from build123d import *

# Parameters (mm, degrees)
SKETCH_1_R      = 1.75
SKETCH_1_W      = 3
SKETCH_1_H      = 8
SKETCH_1_W_2    = 41
SKETCH_1_H_2    = 11
EXTRUDE_1_DEPTH = 5


with BuildPart() as part:
    # Эскиз1 → Бобышка-Вытянуть1 (new body)
    with BuildSketch(Plane(origin=(0, 0, 0), x_dir=(0, 0, -1), z_dir=(1, 0, 0))):
        with BuildLine():
            Line((-36.75, 45), (-36.75, 42.5))
            Line((-36.75, 42.5), (-39.25, 42.5))
            Line((-39.25, 42.5), (-39.25, 40))
            Line((-39.25, 40), (-30.75, 40))
            Line((-30.75, 40), (-30.75, 42.5))
            Line((-30.75, 42.5), (-33.25, 42.5))
            Line((-33.25, 42.5), (-33.25, 45))
            Line((-33.25, 45), (33.25, 45))
            Line((33.25, 45), (33.25, 42.5))
            Line((33.25, 42.5), (30.75, 42.5))
            Line((30.75, 42.5), (30.75, 40))
            Line((30.75, 40), (39.25, 40))
            Line((39.25, 40), (39.25, 42.5))
            Line((39.25, 42.5), (36.75, 42.5))
            Line((36.75, 42.5), (36.75, 45))
            Line((36.75, 45), (43, 45))
            ThreePointArc((43, 45), (44.414213562, 44.414213562), (45, 43))
            Line((45, 43), (45, 31.75))
            Line((45, 31.75), (42.5, 31.75))
            Line((42.5, 31.75), (42.5, 34.25))
            Line((42.5, 34.25), (40, 34.25))
            Line((40, 34.25), (40, 25.75))
            Line((40, 25.75), (42.5, 25.75))
            Line((42.5, 25.75), (42.5, 28.25))
            Line((42.5, 28.25), (45, 28.25))
            Line((45, 28.25), (45, -28.25))
            Line((45, -28.25), (42.5, -28.25))
            Line((42.5, -28.25), (42.5, -25.75))
            Line((42.5, -25.75), (40, -25.75))
            Line((40, -25.75), (40, -34.25))
            Line((40, -34.25), (42.5, -34.25))
            Line((42.5, -34.25), (42.5, -31.75))
            Line((42.5, -31.75), (45, -31.75))
            Line((45, -31.75), (45, -43))
            ThreePointArc((45, -43), (44.414213562, -44.414213562), (43, -45))
            Line((43, -45), (36.75, -45))
            Line((36.75, -45), (36.75, -42.5))
            Line((36.75, -42.5), (39.25, -42.5))
            Line((39.25, -42.5), (39.25, -40))
            Line((39.25, -40), (30.75, -40))
            Line((30.75, -40), (30.75, -42.5))
            Line((30.75, -42.5), (33.25, -42.5))
            Line((33.25, -42.5), (33.25, -45))
            Line((33.25, -45), (-33.25, -45))
            Line((-33.25, -45), (-33.25, -42.5))
            Line((-33.25, -42.5), (-30.75, -42.5))
            Line((-30.75, -42.5), (-30.75, -40))
            Line((-30.75, -40), (-39.25, -40))
            Line((-39.25, -40), (-39.25, -42.5))
            Line((-39.25, -42.5), (-36.75, -42.5))
            Line((-36.75, -42.5), (-36.75, -45))
            Line((-36.75, -45), (-43, -45))
            ThreePointArc((-43, -45), (-44.414213562, -44.414213562), (-45, -43))
            Line((-45, -43), (-45, -31.75))
            Line((-45, -31.75), (-42.5, -31.75))
            Line((-42.5, -31.75), (-42.5, -34.25))
            Line((-42.5, -34.25), (-40, -34.25))
            Line((-40, -34.25), (-40, -25.75))
            Line((-40, -25.75), (-42.5, -25.75))
            Line((-42.5, -25.75), (-42.5, -28.25))
            Line((-42.5, -28.25), (-45, -28.25))
            Line((-45, -28.25), (-45, 28.25))
            Line((-45, 28.25), (-42.5, 28.25))
            Line((-42.5, 28.25), (-42.5, 25.75))
            Line((-42.5, 25.75), (-40, 25.75))
            Line((-40, 25.75), (-40, 34.25))
            Line((-40, 34.25), (-42.5, 34.25))
            Line((-42.5, 34.25), (-42.5, 31.75))
            Line((-42.5, 31.75), (-45, 31.75))
            Line((-45, 31.75), (-45, 43))
            ThreePointArc((-45, 43), (-44.414213562, 44.414213562), (-43, 45))
            Line((-43, 45), (-36.75, 45))
        make_face()
        with Locations((-30, -22.5)):
            Circle(SKETCH_1_R, mode=Mode.SUBTRACT)
        with Locations((30, -22.5)):
            Circle(SKETCH_1_R, mode=Mode.SUBTRACT)
        with Locations((8.5, -10)):
            Rectangle(SKETCH_1_W, SKETCH_1_H, mode=Mode.SUBTRACT)
        with Locations((-8.5, -10)):
            Rectangle(SKETCH_1_W, SKETCH_1_H, mode=Mode.SUBTRACT)
        with Locations((4.5, 14.5)):
            Rectangle(SKETCH_1_W_2, SKETCH_1_H_2, mode=Mode.SUBTRACT)
    extrude(amount=EXTRUDE_1_DEPTH)


solid = part.part
Work out the finished part from the listing and answer in its coordinate system (mm). A direction names the side the tool comes from. Give positions to 0.01 mm unless a question says otherwise; leave off trailing zeros. Order: outer loops, then holes, each group sorted by start corner. A loop starts at its lowest first (then second) coordinate and runs counter-clockwise, first axis right, second up. Notation, with made-up numbers: (-6.5, -13.75) - (5.5, -13.75) arc R16 cw to (5.5, -1.75) - close; hole circle Ø5 at (58.25, 10). An arc over 180 degrees is marked (long way). Answer as CSV lines item,"result". Start each with the question number.
Q1. Find the intervals of material crossed by L1, parallel to Z at x = 1.3, y = -13.5; L2, parallel to Z at x = 0.55, y = 33.5, in increasing order. Write a range as [from, to].
Q2. For faces 4 (the face through (2, 44, 36.75)), 5 (the face through (2, 31.75, -44)), 6 (the face through (2, -44, 33.25)), 7 (the face through (2, 14, 16)), determine the directions among +Z, -Z, +X, -X, +Y, -Y from which every point of the face is accessible in a straight line to the end or side of a thin tool.
Q3. The part is cut by section D-D (y = 30). Write down the section's boundary in (x, z), then the cut area to 3 significant figures.
Q4. The part is cut by section B-B (z = -18.5). Write down the section's boundary in (x, y).
Q5. The part is cut by section C-C (x = 1.2). Give the number of separate pieces and of enclosed holes in the cut face, then the cut area to 3 significant figures.
Q6. The part is cut by section A-A (y = -22.5). Write down the section's boundary in (x, z), then the cut area to 3 significant figures.
Q7. The mould has two halves that part along Y. Classify faces 1 (the face through (2, 45, 40)), 2 (the face through (2, -25.75, 41)), 3 (the face through (2, 0, 45)): +Y half, -Y half, draft (parallel to the pull), parting line (faces both ways), or undercut.
Check result:
1,L1,"z = [-45, -10], [-7, 7], [10, 45]"
1,L2,"z = [-45, -42.5], [-40, 40], [42.5, 45]"
2,face 4,"+X, -X, +Y"
2,face 5,"-Z, +X, -X"
2,face 6,"+X, -X, -Y"
2,face 7,"+X, -X"
3,outline,"(0, -40) - (5, -40) - (5, 40) - (0, 40) - close"
3,area,"400 mm²"
4,outline,"(0, -45) - (5, -45) - (5, 9) - (0, 9) - close; (0, 20) - (5, 20) - (5, 45) - (0, 45) - close"
5,separate pieces,"1"
5,enclosed holes,"5"
5,area,"7,340 mm²"
6,outline,"(0, -45) - (5, -45) - (5, -31.75) - (0, -31.75) - close; (0, -28.25) - (5, -28.25) - (5, 28.25) - (0, 28.25) - close; (0, 31.75) - (5, 31.75) - (5, 45) - (0, 45) - close"
6,area,"415 mm²"
7,face 1,"+Y half"
7,face 2,"undercut"
7,face 3,"draft"
